The figure shows three views and two pictorial views of one solid part (mm, origin at its lowest corner). Answer the questions. A direction names the side the tool comes from. Coordinates: 2 decimals unless noted, no trailing zeros. Loops run counter-clockwise (first coordinate to the right, second up) from the corner with the lowest first, then second, coordinate; pieces in that order, holes last.
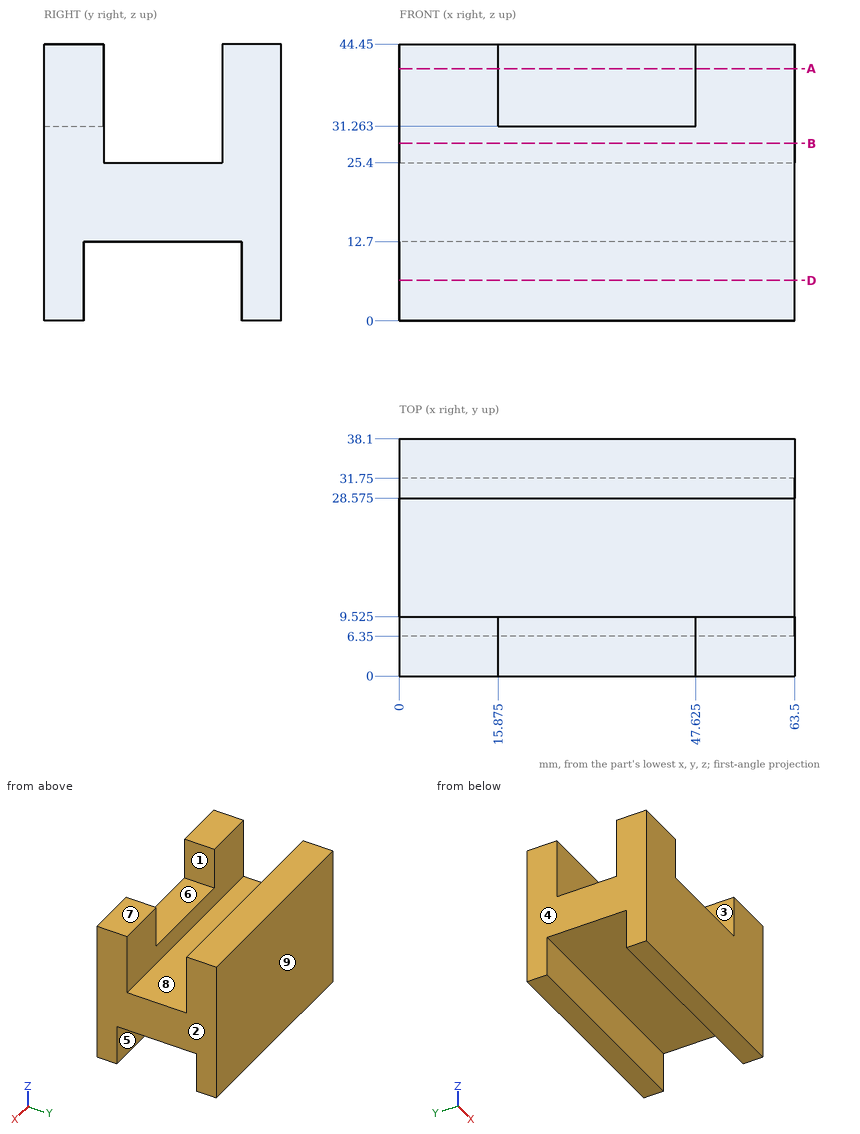
1. A cutting plane is placed at D-D, the plane z = 6.5. Give the vertices of the cut face in (x, y).
2. Straight lines are drawn through the part: probe 1 along Y at (x, z) = (54.5, 41) (3 decimals); probe 2 along Y at (x, z) = (18.5, 7); probe 3 along X at (y, z) = (5, 36) (3 decimals). For each, find the intervals that lie inside material, in ascending order.
3. A cutting plane is placed at A-A, the plane z = 40.5. Give the vertices of the cut face in (x, y) (3 decimals), then the cut area to 3 significant figures.
4. A cutting plane is placed at B-B, the plane z = 28.5. Give the vertices of the cut face in (x, y) (3 decimals).
5. Each of these flat-tipped pins is pushed along its axis until it touches: P1, Ø5, axis at x = 28, z = 21, coming from the -Y side; P2, Ø6, axis at x = 32, y = 10.5, coming from the +Z side; P3, Ø1.5, axis at x = 39, y = 17.5, coming from the +Z side; P4, Ø5.5, axis at x = 42.5, z = 37, coming from the -Y side (3 decimals). Where does it stop, or does it pass through?
6. Determine the mould class of the marked faces 1, 2, 3 and 4 for opening direction X: released by +X, released by -X, zero draft, split by the parting line, or undercut.
7. For the marked faces 5, 6, 7, 8 and 9, determine the directions among +Z, -Z, +X, -X, +Y, -Y from which every point of the face is accessible in a straight line to the end or side of a thin tool.
Answers below:
1. outline: (0, 0) - (63.5, 0) - (63.5, 6.35) - (0, 6.35) - close; (0, 31.75) - (63.5, 31.75) - (63.5, 38.1) - (0, 38.1) - close
2. probe 1: y = 0 to 9.525, 28.575 to 38.1
2. probe 2: y = 0 to 6.35, 31.75 to 38.1
2. probe 3: x = 0 to 15.875, 47.625 to 63.5
3. outline: (0, 0) - (15.875, 0) - (15.875, 9.525) - (0, 9.525) - close; (0, 28.575) - (63.5, 28.575) - (63.5, 38.1) - (0, 38.1) - close; (47.625, 0) - (63.5, 0) - (63.5, 9.525) - (47.625, 9.525) - close
3. area: 907 mm2
4. outline: (0, 0) - (63.5, 0) - (63.5, 9.525) - (0, 9.525) - close; (0, 28.575) - (63.5, 28.575) - (63.5, 38.1) - (0, 38.1) - close
5. P1: stops at y = 0
5. P2: stops at z = 31.26
5. P3: stops at z = 25.4
5. P4: stops at y = 28.575
6. face 1: undercut
6. face 2: released by +X
6. face 3: undercut
6. face 4: released by -X
7. face 5: -Z, +X, -X
7. face 6: +Z, -Y
7. face 7: +Z, +X, -X, +Y, -Y
7. face 8: +Z, +X, -X
7. face 9: +Z, -Z, +X, -X, +Y
